Autodesk Inventor part; units mm, degrees
ref_plane "XY Plane" through (0, 0, 0) normal (0, 0, 1) x (1, 0, 0)
sketch "Skizze1" plane through (0, 0, 0) normal (0, 0, 1) x (1, 0, 0)
  circle A0 centre (0, 0) radius 30
  dimension "d0" = 60
extrude "Extrusion1" add sketch "Skizze1" along normal blind 10
sketch "Skizze2" plane through (0, 0, 10) normal (0, 0, 1) x (1, 0, 0)
  circle A0 centre (0, 0) radius 30
  circle A1 centre (0, 0) radius 24
  circle A2 centre (0, 0) radius 3
  dimension "d3" = 6
  dimension "d4" = 6
extrude "Extrusion2" cut sketch "Skizze2" against normal blind 7 contours A1 | A2
sketch "Skizze3" plane through (0, 0, 10) normal (0, 0, 1) x (1, 0, 0)
  circle A0 centre (0, 0) radius 3.5
  dimension "d7" = 7
extrude "Extrusion3" cut sketch "Skizze3" along normal through all both and the other way through all
fillet "Rundung1" radius 0.2 1 edges at (-24, 0, 3)
chamfer "Fase1" distance 0.2 angle 45 3 edges at (-30, 0, 0) (-30, 0, 10) (-24, 0, 10)
sketch "Skizze4" plane through (0, 0, 10) normal (0, 0, 1) x (1, 0, 0)
  circle A0 centre (0, 0) radius 27
  circle A1 centre (0, 0) radius 37
  dimension "d14" = 54
  dimension "d15" = 10
extrude "Extrusion4" cut sketch "Skizze4" along normal through all both and the other way through all
ref_plane "Arbeitsebene1" through (22.5, 0, 0) normal (1, 0, 0) x (0, 1, 0)
ref_plane "Arbeitsebene2" through (0, 0, 0) normal (0, 1, 0) x (-1, 0, 0)
hole "Bohrung2" at (22.5, 0, 0) direction (0, 0, 1) diameter 3 depth 3 tip angle 118
pattern_circular "Runde Anordnung2" count 2 over 360 about axis through (0, 0, 10) along (0, 0, 1) of "Bohrung2"
sketch "Skizze6" plane through (0, 0, 10) normal (0, 0, 1) x (1, 0, 0)
  circle A0 centre (-22.5, 0) radius 1.5
  circle A1 centre (0, 0) radius 24.2
  dimension "d25" = 3
  dimension "d26" = 22.5
sketch "Skizze5" plane through (0, 0, 10) normal (0, 0, 1) x (1, 0, 0)
  circle A0 centre (0, 0) radius 3.2
  circle A1 centre (0, 0) radius 27.5
  circle A2 centre (0, 0) radius 30
  dimension "d18" = 55
  dimension "d19" = 60
properties part number "felge" material "Aluminium 6061"
The listing builds one solid part. Answer for the finished solid, in the listing's coordinates (mm). A direction names the side the tool comes from. Round coordinates to 2 decimals unless told otherwise and drop trailing zeros. Loops run counter-clockwise (first coordinate to the right, second up) from the corner with the lowest first, then second, coordinate; pieces in that order, holes last.
1) A cutting plane is placed at B-B on z = 6.5. Determine the outline of the cut face in (x, y), plus the area to 3 significant figures.
Outcome:
outline: circle Ø54 at (0, 0); hole circle Ø48 at (0, 0)
area: 481 mm2
2) Consider line 1 (Y direction, x = 0, z = 2); line 2 (Y direction, x = 0, z = 8); line 3 (Z direction, x = 14, y = 9.5). Determine where each line is inside the solid, lowest interval first.
Outcome:
line 1: y = -27 to -3.5, 3.5 to 27
line 2: y = -27 to -24, 24 to 27
line 3: z = 0 to 3
3) A cutting plane is placed at A-A on y = 0. Determine the outline of the cut face in (x, z), plus the area to 3 significant figures.
Outcome:
outline: (-27, 0) - (-24, 0) - (-24, 3) - (-23.93, 3.04) arc R0.2 cw to (-24, 3.2) - (-24, 9.8) - (-24.2, 10) - (-27, 10) - close; (-21, 0) - (-3.5, 0) - (-3.5, 3) - (-21, 3) - close; (3.5, 0) - (21, 0) - (21, 3) - (3.5, 3) - close; (23.93, 3.04) - (24, 3) - (24, 0) - (27, 0) - (27, 10) - (24.2, 10) - (24, 9.8) - (24, 3.2) arc R0.2 cw to start
area: 165 mm2
4) Given P1, Ø2.5, axis at x = 22.5, y = 0, coming from the +Z side; P2, Ø6, axis at y = -9, z = 8.5, coming from the +X side; P3, Ø1, axis at x = -19, z = 7, coming from the +Y side; P4, Ø1.5, axis at x = 13.5, z = 8, coming from the +Y side, each flat-ended and moving along its own axis, determine where each tip first touches the part or whether it passes through.
Outcome:
P1: passes through
P2: stops at x = 26.32
P3: stops at y = 19.67
P4: stops at y = 23.8
5) For a pull along X with two mould halves and no side action, classify faces 1 (the face through (21, 0, 2)), 2 (the face through (-4.1, 24.1, 10)), 3 (the face through (-5.85, -26.36, 5.07)), 4 (the face through (-21, 0, 2)) as released by +X, released by -X, zero draft, split by the parting line, or undercut.
Outcome:
face 1: undercut
face 2: zero draft
face 3: split by the parting line
face 4: undercut
6) For faces 5 (the face through (3.233, -1.341, 1.521)), 6 (the face through (-23.977, 1.055, 6.546)), determine the directions among +Z, -Z, +X, -X, +Y, -Y from which every point of the face is accessible in a straight line to the end or side of a thin tool.
Outcome:
face 5: +Z, -Z
face 6: +Z
